```python
from build123d import *

# Parameters (mm, degrees)
F0_W     = 150
F0_H     = 150
F1_DEPTH = 600
F2_R     = 10
F3_R     = 15
F4_DEPTH = 50


with BuildPart() as f1:
    # F0 (on Top) → F1 (new body)
    with BuildSketch(Plane.XY):
        with Locations((75, 75)):
            Rectangle(F0_W, F0_H)
    extrude(amount=F1_DEPTH)

    # F2
    f2_edges = [f1.edges().sort_by_distance(p)[0] for p in [
        (0, 150, 300),
        (150, 150, 300),
        (150, 0, 300),
        (0, 0, 300),
    ]]
    fillet(f2_edges, radius=F2_R)

    # F3 (on face) → F4 (cut)
    with BuildSketch(Plane.XY.offset(600)):
        with Locations((50, 100)):
            Circle(F3_R)
        with Locations((100, 100)):
            Circle(F3_R)
        with Locations((100, 50)):
            Circle(F3_R)
        with Locations((50, 50)):
            Circle(F3_R)
    extrude(amount=-F4_DEPTH, mode=Mode.SUBTRACT)


solid = f1.part
```
The listing builds one solid part. Answer for the finished solid, in the listing's coordinates (mm). A direction names the side the tool comes from. Give positions to 0.01 mm unless a question says otherwise; leave off trailing zeros. Order: outer loops, then holes, each group sorted by start corner. A loop starts at its lowest first (then second) coordinate and runs counter-clockwise, first axis right, second up. Notation, with made-up numbers: (30.5, 77) -> (60.5, 77) arc R24 cw to (60.5, 103) -> close; hole circle Ø10 at (-0.5, 31.5). An arc over 180 degrees is marked (long way). One line per item, written item: value.
1) A flat-ended cylindrical pin translates along its axis: P1, Ø9, axis at x = 100, y = 95.5, coming from the +Z side. Find the tip coordinate at first contact, or state that the pin passes through.
Reported:
P1: stops at z = 550
2) Determine the mould class of faces 3 (the flat face through (150, 74, 296)), 4 (the flat face through (100, 50, 550)), 5 (the cylindrical face through (2.85, 3.01, 304.2)) for opening direction X: pulls with the +X half, pulls with the -X half, needs draft (parallel to the pull), parting line crosses it, or undercut.
Reported:
face 3: pulls with the +X half
face 4: undercut
face 5: pulls with the -X half
3) Find the intervals of material crossed by line 1 (Y direction, x = 100, z = 583.5); line 2 (Z direction, x = 38, y = 107), in increasing order.
Reported:
line 1: y = 0 to 35, 65 to 85, 115 to 150
line 2: z = 0 to 550
4) A tool of negligible diameter and unlimited length cuts with its end or side. For faces 1 (the cylindrical face through (46.748, 85.357, 575.35)), 2 (the flat face through (74, 150, 296)), from which of +Z, -Z, +X, -X, +Y, -Y can it reach the whole face along a straight path? Write none if from no direction.
Reported:
face 1: +Z
face 2: +Z, -Z, +X, -X, +Y
5) Find section A-A, the plane y = 100. Determine the outline of the cut face in (x, z).
Reported:
outline: (0, 0) -> (150, 0) -> (150, 600) -> (115, 600) -> (115, 550) -> (85, 550) -> (85, 600) -> (65, 600) -> (65, 550) -> (35, 550) -> (35, 600) -> (0, 600) -> close
